from build123d import *

# Parameters (mm, degrees)
SKETCH1_R           = 6.273243026
SKETCH1_R_2         = 1.25
BOSS_EXTRUDE1_DEPTH = 3.2
BOSS_EXTRUDE2_DEPTH = 50
CUT_EXTRUDE1_REACH  = 78.812
SKETCH3_R           = 2


with BuildPart() as part:
    # Sketch1 → Boss-Extrude1 (new body)
    with BuildSketch(Plane.XY):
        with BuildLine():
            Line((-25, 0), (-25, 30))
            Line((-25, 30), (25, 30))
            Line((25, 30), (25, 0))
            ThreePointArc((25, 0), (0, -25), (-25, 0))
        make_face()
        Circle(SKETCH1_R, mode=Mode.SUBTRACT)
        with Locations((0, 11)):
            Circle(SKETCH1_R_2, mode=Mode.SUBTRACT)
        with Locations((9.526279442, -5.5)):
            Circle(SKETCH1_R_2, mode=Mode.SUBTRACT)
        with Locations((-9.526279442, -5.5)):
            Circle(SKETCH1_R_2, mode=Mode.SUBTRACT)
    extrude(amount=BOSS_EXTRUDE1_DEPTH)

    # Sketch2 → Boss-Extrude2 (add)
    with BuildSketch(Plane(origin=(25, 0, 0), x_dir=(0, 0, -1), z_dir=(1, 0, 0))):
        Polygon((0, 30), (51.961524227, 60), (50.361524227, 62.771281292), (-3.2, 31.847520861), (-3.2, 30), align=None)
    extrude(amount=-BOSS_EXTRUDE2_DEPTH)

    # Sketch3 → Cut-Extrude1 (cut, up to next)
    with BuildSketch(Plane(origin=(0, 25.271281292, 14.590381057), x_dir=(1, 0, 0), z_dir=(0, 0.866025404, 0.5)), mode=Mode.PRIVATE) as cut_extrude1_sk1:
        with Locations((15, 59.076239569)):
            Circle(SKETCH3_R)
    cut_extrude1_tool1 = extrude(cut_extrude1_sk1.sketch, amount=-CUT_EXTRUDE1_REACH, mode=Mode.PRIVATE) & part.part
    add(cut_extrude1_tool1.solids().sort_by_distance((15, 54.809401, -36.571143))[0], mode=Mode.SUBTRACT)
    # Sketch3 → Cut-Extrude1 (cut, up to next)
    with BuildSketch(Plane(origin=(0, 25.271281292, 14.590381057), x_dir=(1, 0, 0), z_dir=(0, 0.866025404, 0.5)), mode=Mode.PRIVATE) as cut_extrude1_sk2:
        with Locations((15, 29.076239569)):
            Circle(SKETCH3_R)
    cut_extrude1_tool2 = extrude(cut_extrude1_sk2.sketch, amount=-CUT_EXTRUDE1_REACH, mode=Mode.PRIVATE) & part.part
    add(cut_extrude1_tool2.solids().sort_by_distance((15, 39.809401, -10.590381))[0], mode=Mode.SUBTRACT)
    # Sketch3 → Cut-Extrude1 (cut, up to next)
    with BuildSketch(Plane(origin=(0, 25.271281292, 14.590381057), x_dir=(1, 0, 0), z_dir=(0, 0.866025404, 0.5)), mode=Mode.PRIVATE) as cut_extrude1_sk3:
        with Locations((-15, 59.076239569)):
            Circle(SKETCH3_R)
    cut_extrude1_tool3 = extrude(cut_extrude1_sk3.sketch, amount=-CUT_EXTRUDE1_REACH, mode=Mode.PRIVATE) & part.part
    add(cut_extrude1_tool3.solids().sort_by_distance((-15, 54.809401, -36.571143))[0], mode=Mode.SUBTRACT)
    # Sketch3 → Cut-Extrude1 (cut, up to next)
    with BuildSketch(Plane(origin=(0, 25.271281292, 14.590381057), x_dir=(1, 0, 0), z_dir=(0, 0.866025404, 0.5)), mode=Mode.PRIVATE) as cut_extrude1_sk4:
        with Locations((-15, 29.076239569)):
            Circle(SKETCH3_R)
    cut_extrude1_tool4 = extrude(cut_extrude1_sk4.sketch, amount=-CUT_EXTRUDE1_REACH, mode=Mode.PRIVATE) & part.part
    add(cut_extrude1_tool4.solids().sort_by_distance((-15, 39.809401, -10.590381))[0], mode=Mode.SUBTRACT)


solid = part.part
Can you work these out from the model? Positions are in its coordinate system, mm. A direction names the side the tool comes from. Give positions to 0.01 mm unless a question says otherwise; leave off trailing zeros. Order: outer loops, then holes, each group sorted by start corner. A loop starts at its lowest first (then second) coordinate and runs counter-clockwise, first axis right, second up. Notation, with made-up numbers: M 61,20.5 L 66,20.5 A33 cw 66,58.5 Z; hole C 61.5,3 d3. An arc over 180 degrees is marked long. Use a Markdown table: item, result. Add a question column.
Item 1: Suppose I cut it at D-D (y = 23). List the corners of the cut face in (x, z) for me.
Item 2: Suppose I cut it at A-A (y = 11). List the corners of the cut face in (x, z) for me, then the cut area to 3 significant figures.
Item 3: Suppose I cut it at C-C (x = -20.5). List the corners of the cut face in (y, z) for me, then the cut area to 3 significant figures.
Item 4: Will these pins go through, and if not, where does the flat tip stop? pin 1 (3 mm diameter, centred on x = 5, y = 24, fed in from -Z); pin 2 (2 mm diameter, centred on x = 0, y = 11, fed in from -Z); pin 3 (3 mm diameter, centred on x = -1.5, z = -28, fed in from -Y); pin 4 (3 mm diameter, centred on x = 7, z = -42, fed in from -Y).
Item 5: For faces 5 (the flat face through (0, 9, 0)), 6 (the flat face through (0.35, 47.53, -23.96)), which set-ups out of +Z, -Z, +X, -X, +Y, -Y let a thin tool reach every point of the face, with its end or its side?
Item 6: If I drill on L1, parallel to Y at x = 0, z = 0.7; L2, parallel to Y at x = 0, z = 2.1; L3, parallel to Z at x = 10, y = 17, over which ranges is the centre line in solid material (lowest first)? Write a range as [from, to].
Item 7: We'd pull the mould along X, two halves only. Please class faces 1 (the flat face through (0.35, 44.79, -25.62)), 2 (the cylindrical face through (-0.16, 12.24, 1.58)), 3 (the flat face through (25, 39, -14)), 4 (the cylindrical face through (5.795, -2.403, 1.578)): +X half, -X half, draft (parallel to the pull), parting line (faces both ways), or undercut.
Item 8: Suppose I cut it at B-B (x = -15.5). List the corners of the cut face in (y, z) for me, then the cut area to 3 significant figures.
Answer sheet:
| question | item | result |
|---|---|---|
| 1 | outline | M -25,0 L 25,0 L 25,3.2 L -25,3.2 Z |
| 2 | outline | M -25,0 L -1.25,0 L -1.25,3.2 L -25,3.2 Z; M 1.25,0 L 25,0 L 25,3.2 L 1.25,3.2 Z |
| 2 | area | 152 mm² |
| 3 | outline | M -14.31,0 L 30,0 L 60,-51.96 L 62.77,-50.36 L 31.85,3.2 L -14.31,3.2 Z |
| 3 | area | 340 mm² |
| 4 | pin 1 | stops at z = 0 |
| 4 | pin 2 | passes through |
| 4 | pin 3 | stops at y = 45.3 |
| 4 | pin 4 | stops at y = 53.38 |
| 5 | face 5 | -Z, +X, -X, -Y |
| 5 | face 6 | +Z, +X, -X, +Y |
| 6 | L1 | y = [-25, -6.27], [6.27, 9.75], [12.25, 33.29] |
| 6 | L2 | y = [-25, -6.27], [6.27, 9.75], [12.25, 32.48] |
| 6 | L3 | z = [0, 3.2] |
| 7 | face 1 | draft |
| 7 | face 2 | undercut |
| 7 | face 3 | +X half |
| 7 | face 4 | undercut |
| 8 | outline | M -19.62,0 L 30,0 L 36.07,-10.51 L 38.84,-8.91 L 31.85,3.2 L -19.62,3.2 Z; M 38.01,-13.87 L 51.07,-36.49 L 53.84,-34.89 L 40.78,-12.27 Z; M 53.01,-39.85 L 60,-51.96 L 62.77,-50.36 L 55.78,-38.25 Z |
| 8 | area | 332 mm² |
